Input: part model. Units: mm. Frame: model coordinates. A direction names the side the tool comes from. Round coordinates to 2 decimals unless told otherwise and drop trailing zeros. Loops run counter-clockwise (first coordinate to the right, second up) from the corner with the lowest first, then second, coordinate; pieces in that order, holes last. Notation, with made-up numbers: (34, -28) - (88, -28) arc R24 ccw to (88, 2) - close; hole circle Ø11 at (11, 80). An arc over 180 degrees is marked (long way). Use CSV: the item, a comma, the result in double quotes. Start each with the question number.
1. Cut plane A-A (y = 0). Return loops of the section in (x, z), and give its area (3 significant figures).
2. Pin query (flat end, axial travel): P1, Ø2, axis at x = 54.19, y = -8.8, coming from the +Z side; P2, Ø23.5, axis at x = -16, y = 11, coming from the +Z side; P3, Ø20, axis at x = -0.5, y = -4.5, coming from the -Z side. Return the tip coordinate at first contact, or that it passes through.
3. Material intervals for probe 1 along X at (y, z) = (8, -20); probe 2 along X at (y, z) = (4, -17); probe 3 along Y at (x, z) = (-9, -27), sorted ascending. Write a range as from..to.
4. Access query for faces 4 (the flat face through (-1, 1, -10)), 5 (the flat face through (0, 25, -25)), 6 (the flat face through (-1, 75, -17)). Directions: +Z, -Z, +X, -X, +Y, -Y. A direction counts if a zero-diameter tool reaches every point of the face in a straight line with its end or side. Return the directions, or none.
5. Cut plane B-B (z = -21). Return loops of the section in (x, y), and give its area (3 significant figures).
6. Cut plane C-C (x = -13). Return loops of the section in (y, z).
7. Pull-direction query (X, two-part tool) for faces 1 (the flat face through (0, -25, -25)), 2 (the flat face through (75, -1, -17)), 3 (the flat face through (-34, 34, 0)); classes: +X half, -X half, draft (parallel to the pull), parting line (faces both ways), or undercut.
8. Cut plane D-D (z = -3.5). Return loops of the section in (x, y).
```python
from build123d import *

# Parameters (mm, degrees)
SKETCH1_W                   = 150
SKETCH1_H                   = 150
BOSS_EXTRUDE1_DEPTH         = 35
FILLET1_R                   = 1
SKETCH2_R                   = 39.25
CUT_EXTRUDE4_DEPTH          = 10
TAP_DRILL_FOR_M3X0_5_TAP2_D = 2.5
TAP_DRILL_FOR_M3X0_5_TAP3_D = 2.5
TAP_DRILL_FOR_M3X0_5_TAP5_D = 2.5
SKETCH31_W                  = 40.1
SKETCH31_H                  = 50
CUT_EXTRUDE5_DEPTH          = 20.3


with BuildPart() as part:
    # Sketch1 → Boss-Extrude1 (new body)
    with BuildSketch(Plane.XY):
        Rectangle(SKETCH1_W, SKETCH1_H)
    extrude(amount=-BOSS_EXTRUDE1_DEPTH)

    # Fillet1
    fillet1_edges = [part.edges().sort_by_distance(p)[0] for p in [
        (0, 75, -35),
        (-75, 0, 0),
        (0, 75, 0),
        (75, 0, 0),
        (0, -75, 0),
        (-75, -75, -17.5),
        (-75, 75, -17.5),
        (75, 75, -17.5),
        (75, -75, -17.5),
        (75, 0, -35),
    ]]
    fillet(fillet1_edges, radius=FILLET1_R)

    # Sketch2 → Cut-Extrude4 (cut)
    with BuildSketch(Plane.XY):
        Circle(SKETCH2_R)
    extrude(amount=-CUT_EXTRUDE4_DEPTH, mode=Mode.SUBTRACT)

    # Tap Drill for M3x0.5 Tap2 (through all)
    with Locations(Plane.XY):
        with Locations((-54.190883488, -8.8), (-54.190883488, 8.8), (54.190883488, -8.8), (54.190883488, 8.8)):
            Hole(TAP_DRILL_FOR_M3X0_5_TAP2_D / 2)

    # Tap Drill for M3x0.5 Tap3 (through all)
    with Locations(Plane.XY):
        with Locations((-49, -11)):
            Hole(TAP_DRILL_FOR_M3X0_5_TAP3_D / 2)

    # Tap Drill for M3x0.5 Tap5 (through all)
    with Locations(Plane.XY):
        with Locations((-0.083892693, -49.999977478)):
            Hole(TAP_DRILL_FOR_M3X0_5_TAP5_D / 2)

    # Sketch31 → Cut-Extrude5 (cut)
    with BuildSketch(Plane(origin=(0, 0, -35), x_dir=(-1, 0, 0), z_dir=(0, 0, -1))):
        Rectangle(SKETCH31_W, SKETCH31_H)
    extrude(amount=-CUT_EXTRUDE5_DEPTH, mode=Mode.SUBTRACT)


solid = part.part
```
Established:
1,outline,"(-75, -35) - (-20.05, -35) - (-20.05, -14.7) - (20.05, -14.7) - (20.05, -35) - (74, -35) arc R1 ccw to (75, -34) - (75, -1) arc R1 ccw to (74, 0) - (39.25, 0) - (39.25, -10) - (-39.25, -10) - (-39.25, 0) - (-74, 0) arc R1 ccw to (-75, -1) - close"
1,area,"3,650 mm2"
2,P1,"passes through"
2,P2,"stops at z = -10"
2,P3,"stops at z = -14.7"
3,probe 1,"x = -75..-55.15, -53.23..-20.05, 20.05..53.23, 55.15..75"
3,probe 2,"x = -75..-20.05, 20.05..75"
3,probe 3,"y = -75..-25, 25..75"
4,face 4,"+Z"
4,face 5,"-Z"
4,face 6,"+Z, -Z, +X, -X, +Y"
5,outline,"(-75, -74) arc R1 ccw to (-74, -75) - (74, -75) arc R1 ccw to (75, -74) - (75, 74) arc R1 ccw to (74, 75) - (-74, 75) arc R1 ccw to (-75, 74) - close; hole circle Ø2.5 at (-54.19, -8.8); hole circle Ø2.5 at (-54.19, 8.8); hole circle Ø2.5 at (-49, -11); hole (-20.05, -25) - (20.05, -25) - (20.05, 25) - (-20.05, 25) - close; hole circle Ø2.5 at (-0.08, -50); hole circle Ø2.5 at (54.19, -8.8); hole circle Ø2.5 at (54.19, 8.8)"
5,area,"20,500 mm2"
6,outline,"(-75, -35) - (-25, -35) - (-25, -14.7) - (25, -14.7) - (25, -35) - (74, -35) arc R1 ccw to (75, -34) - (75, -1) arc R1 ccw to (74, 0) - (37.03, 0) - (37.03, -10) - (-37.03, -10) - (-37.03, 0) - (-74, 0) arc R1 ccw to (-75, -1) - close"
7,face 1,"undercut"
7,face 2,"+X half"
7,face 3,"draft"
8,outline,"(-75, -74) arc R1 ccw to (-74, -75) - (74, -75) arc R1 ccw to (75, -74) - (75, 74) arc R1 ccw to (74, 75) - (-74, 75) arc R1 ccw to (-75, 74) - close; hole circle Ø2.5 at (-54.19, -8.8); hole circle Ø2.5 at (-54.19, 8.8); hole circle Ø2.5 at (-49, -11); hole circle Ø78.5 at (0, 0); hole circle Ø2.5 at (-0.08, -50); hole circle Ø2.5 at (54.19, -8.8); hole circle Ø2.5 at (54.19, 8.8)"
